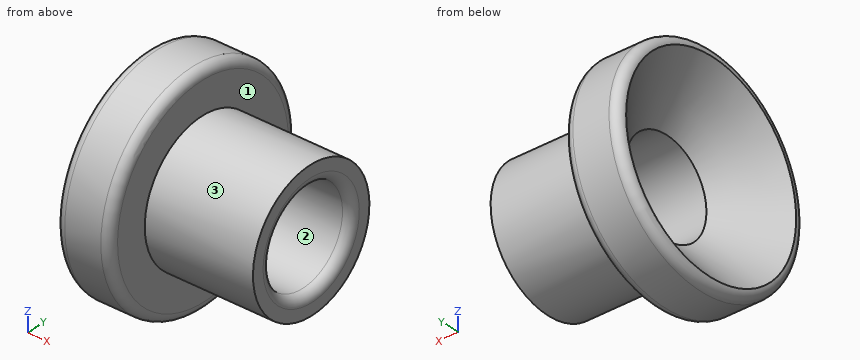
from build123d import *

# Parameters (mm, degrees)
SKETCH1_R           = 7.62
SKETCH1_R_2         = 3.302
BOSS_EXTRUDE1_DEPTH = 3.81
SKETCH2_R           = 4.7625
SKETCH2_R_2         = 3.302
BOSS_EXTRUDE2_DEPTH = 10.795
FILLET1_R           = 0.635
CHAMFER1_SIZE       = 3.175
CHAMFER1_SIZE2      = 3.652419693
CUT_EXTRUDE1_START  = -3.175
SKETCH3_R           = 4.7625
CUT_EXTRUDE1_DEPTH  = 3.175
FILLET2_R           = 0.635


with BuildPart() as part:
    # Sketch1 → Boss-Extrude1 (new body)
    with BuildSketch(Plane(origin=(0, 0, 0), x_dir=(0, 0, -1), z_dir=(1, 0, 0))):
        with Locations(Location((0, 0, 0), (0, 0, 180))):
            Circle(SKETCH1_R)
        with Locations(Location((0, 0, 0), (0, 0, 180))):
            Circle(SKETCH1_R_2, mode=Mode.SUBTRACT)
    extrude(amount=BOSS_EXTRUDE1_DEPTH)

    # Sketch2 → Boss-Extrude2 (add)
    with BuildSketch(Plane(origin=(3.81, 0, 0), x_dir=(0, 0, -1), z_dir=(1, 0, 0))):
        Circle(SKETCH2_R)
        with Locations(Location((0, 0, 0), (0, 0, 180))):
            Circle(SKETCH2_R_2, mode=Mode.SUBTRACT)
    extrude(amount=BOSS_EXTRUDE2_DEPTH)

    # Fillet1
    fillet1_edges = [part.edges().sort_by_distance(p)[0] for p in [
        (14.605, 0, -3.302),
        (0, 0, -7.62),
        (3.81, 0, -7.62),
    ]]
    fillet(fillet1_edges, radius=FILLET1_R)

    # Chamfer1
    chamfer1_edges = [part.edges().sort_by_distance(p)[0] for p in [
        (0, 0, -3.302),
    ]]
    chamfer1_side = [part.faces().sort_by_distance(p)[0] for p in [
        (6.985, 0, -3.302),
    ]]
    chamfer(chamfer1_edges, length=CHAMFER1_SIZE, length2=CHAMFER1_SIZE2, reference=chamfer1_side[0])

    # Sketch3 → Cut-Extrude1 (cut)
    with BuildSketch(Plane(origin=(14.605, 0, 0), x_dir=(0, 0, -1), z_dir=(1, 0, 0)).offset(CUT_EXTRUDE1_START)):
        Circle(SKETCH3_R)
    extrude(amount=CUT_EXTRUDE1_DEPTH, mode=Mode.SUBTRACT)

    # Fillet2
    fillet2_edges = [part.edges().sort_by_distance(p)[0] for p in [
        (11.43, 0, -3.302),
    ]]
    fillet(fillet2_edges, radius=FILLET2_R)


solid = part.part
Source: CAD feature listing. Evaluate the final solid. Frame: model axes, mm. Face numbers are marked on the shaded views. Coordinates: 2 decimals unless noted, no trailing zeros. Loops run counter-clockwise (first coordinate to the right, second up) from the corner with the lowest first, then second, coordinate; pieces in that order, holes last. Notation, with made-up numbers: (23.25, 79.5) -> (38.25, 79.5) arc R28 cw to (38.25, 112.5) -> close; hole circle Ø6 at (66, 36.25). An arc over 180 degrees is marked (long way). Answer in a Markdown table with one row per item. Add a question column.
Q1. Ray query, line 1 along Y through (x, z) = (7, 0); line 2 along Y through (x, z) = (9.5, 1); line 3 along Z through (x, y) = (6.75, -0.5). Return the intervals inside material, ascending.
Q2. Pull-direction query (Z, two-part tool) for the marked faces 1, 2 and 3; classes: pulls with the +Z half, pulls with the -Z half, needs draft (parallel to the pull), parting line crosses it, or undercut.
Q3. Section C-C on x = 5.75. Return the cut outline in (y, z) (1 decimal).
Q4. Contact query for flat-ended pins moving along their axis: pin 1 Ø2 at (y, z) = (-5, -4) entering from +X; pin 2 Ø1 at (x, z) = (8.5, 0.5) entering from -Y; pin 3 Ø3 at (x, y) = (1.5, -3) entering from -Z. Output: stop coordinate, or through.
Computed values:
| question | item | result |
|---|---|---|
| 1 | line 1 | y = -4.76 to -3.3, 3.3 to 4.76 |
| 1 | line 2 | y = -4.66 to -3.15, 3.15 to 4.66 |
| 1 | line 3 | z = -4.74 to -3.26, 3.26 to 4.74 |
| 2 | face 1 | needs draft |
| 2 | face 2 | undercut |
| 2 | face 3 | parting line crosses it |
| 3 | outline | circle Ø9.5 at (0, 0); hole circle Ø6.6 at (0, 0) |
| 4 | pin 1 | stops at x = 3.81 |
| 4 | pin 2 | stops at y = -4.76 |
| 4 | pin 3 | stops at z = -7.47 |
